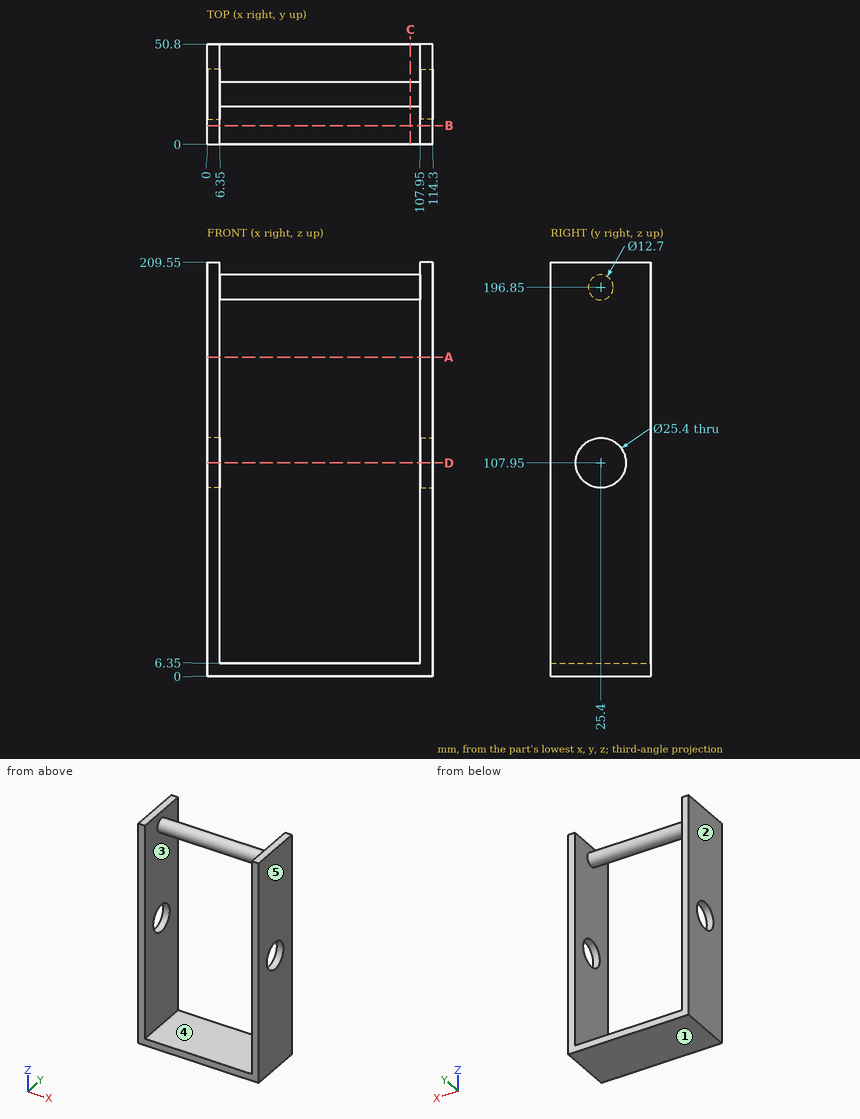
The drawing under review shows one solid part. Ordinate dimensions are in mm from its lowest x, y, z. A direction names the side the tool comes from. Coordinates: 2 decimals unless noted, no trailing zeros. Loops run counter-clockwise (first coordinate to the right, second up) from the corner with the lowest first, then second, coordinate; pieces in that order, holes last. Notation, with made-up numbers: (78, 18.5) - (133, 18.5) arc R20 ccw to (133, 36.5) - close; hole circle Ø11 at (28, 20). An arc over 180 degrees is marked (long way). Return JSON: item names as keys, results as strings.
Item 1: Take a section at A-A (z = 161.5). Give the boundary of the cut face in (x, y).
Determined:
{"outline": "(0, 0) - (6.35, 0) - (6.35, 50.8) - (0, 50.8) - close; (107.95, 0) - (114.3, 0) - (114.3, 50.8) - (107.95, 50.8) - close"}
Item 2: Insertion check: pin 1 (1.5 mm diameter, centred on y = 24, z = 161, fed in from -X); pin 2 (8 mm diameter, centred on x = 31.5, y = 29, fed in from +Z); pin 3 (6 mm diameter, centred on x = 67, y = 8, fed in from +Z); pin 4 (20.5 mm diameter, centred on y = 25.4, z = 107.95, fed in from -X). Each pin has a flat end and moves straight along its axis. Give the tip position at first contact, or say it passes through.
Determined:
{"pin 1": "stops at x = 0", "pin 2": "stops at z = 203.2", "pin 3": "stops at z = 6.35", "pin 4": "passes through"}
Item 3: Take a section at C-C (x = 103). Give the boundary of the cut face in (y, z), then the cut area to 3 significant figures.
Determined:
{"outline": "(0, 0) - (50.8, 0) - (50.8, 6.35) - (0, 6.35) - close; circle Ø12.7 at (25.4, 196.85)", "area": "449 mm2"}
Item 4: For the marked faces 4 and 5, list the 3-axis set-ups (+Z, -Z, +X, -X, +Y, -Y) from which the entire face can be reached by the end or side of a thin tool; tool diameter is ignored.
Determined:
{"face 4": "+Y, -Y", "face 5": "+Z, -Z, +X, +Y, -Y"}
Item 5: Take a section at B-B (y = 9.5). Give the boundary of the cut face in (x, z), then the cut area to 3 significant figures.
Determined:
{"outline": "(0, 0) - (114.3, 0) - (114.3, 209.55) - (107.95, 209.55) - (107.95, 6.35) - (6.35, 6.35) - (6.35, 209.55) - (0, 209.55) - close", "area": "3,310 mm2"}
Item 6: Take a section at D-D (z = 107.95). Give the boundary of the cut face in (x, y), then the cut area to 3 significant figures.
Determined:
{"outline": "(0, 0) - (6.35, 0) - (6.35, 12.7) - (0, 12.7) - close; (0, 38.1) - (6.35, 38.1) - (6.35, 50.8) - (0, 50.8) - close; (107.95, 0) - (114.3, 0) - (114.3, 12.7) - (107.95, 12.7) - close; (107.95, 38.1) - (114.3, 38.1) - (114.3, 50.8) - (107.95, 50.8) - close", "area": "323 mm2"}
Item 7: Mouldability with a two-part tool opening along Z and no side actions: class the marked faces 1, 2 and 3 as pulls with the +Z half, pulls with the -Z half, needs draft (parallel to the pull), parting line crosses it, or undercut.
Determined:
{"face 1": "pulls with the -Z half", "face 2": "needs draft", "face 3": "undercut"}
Item 8: For line 1 (X direction, y = 12.5, z = 113); line 2 (Z direction, x = 109, y = 25); line 3 (Z direction, x = 67.5, y = 39), list the stretches that pass through material, from the lowest coordinate up.
Determined:
{"line 1": "x = 0 to 6.35, 107.95 to 114.3", "line 2": "z = 0 to 95.26, 120.64 to 209.55", "line 3": "z = 0 to 6.35"}
